Input: part model. Units: mm. Frame: model coordinates. A direction names the side the tool comes from. Give positions to 0.01 mm unless a question says otherwise; leave off trailing zeros. Order: outer loops, then holes, each group sorted by start corner. A loop starts at its lowest first (then second) coordinate and runs counter-clockwise, first axis right, second up. Notation, with made-up numbers: (0.25, -17.75) - (11.25, -17.75) arc R11 cw to (11.25, -4.75) - close; hole circle Ø11 at (-13.5, 57.5). An arc over 180 degrees is marked (long way). Answer in a Markdown table with one row per item. Add a question column.
1. Contact query for flat-ended pins moving along their axis: pin 1 (0.6 mm diameter, centred on y = 0, z = -7.5, fed in from +X); pin 2 (1.5 mm diameter, centred on x = 14.5, y = 0, fed in from -Z); pin 3 (0.9 mm diameter, centred on y = 0.5, z = -8, fed in from -X). Output: stop coordinate, or through.
2. Ray query, line 1 (X direction, y = 0.2, z = 11); line 2 (X direction, y = -0.25, z = -9); line 3 (Z direction, x = 16, y = 1.5). Return the intervals inside material, ascending. Write a range as [from, to].
3. Section query A-A on x = 0. Return loops of the section in (y, z).
4. Section query C-C on z = 9.75. Return loops of the section in (x, y).
5. Section query B-B on z = -2.25. Return loops of the section in (x, y), and give its area (3 significant figures).
6. Access query for faces 1 (the face through (20.237, 0, 3)), 2 (the face through (15, 0, -6.915)), 3 (the face through (-10.193, 0, -8)). Directions: +Z, -Z, +X, -X, +Y, -Y. A direction counts if a zero-diameter tool reaches every point of the face in a straight line with its end or side. Return the directions, or none.
7. Section query D-D on x = -13. Return loops of the section in (y, z).
8. Mould query, pull axis X, two halves, no side actions, for faces 4 (the face through (13.72, -0.04, 10.31)), 5 (the face through (-10.743, -0.035, 10.451)), 6 (the face through (-15, 0, -7.195)), 7 (the face through (10.237, 0, -8)). Classes: released by +X, released by -X, zero draft, split by the parting line, or undercut.
```python
from build123d import *

# Parameters (mm, degrees)
CROQUIS1_R              = 9.8
CROQUIS1_R_2            = 1.61
CROQUIS1_R_3            = 1.610199264
CROQUIS1_R_4            = 1.610298895
SALIENTE_EXTRUIR3_DEPTH = 2.5
REDONDEO1_SIZE          = 3
REDONDEO2_SIZE          = 3


with BuildPart() as part:
    # Croquis1 → Saliente-Extruir3 (new, symmetric)
    with BuildSketch(Plane(origin=(0, 0, 0), x_dir=(1, 0, 0), z_dir=(0, 1, 0))):
        Polygon((-20.192989013, 7.194690523), (-10.192989013, 7.194690523), (-10.192989013, 11.914690523), (10.237010987, 11.914690523), (10.237010987, 6.914690523), (20.237010987, 6.914690523), (20.237010987, -12.805309477), (-20.192989013, -12.805309477), align=None)
        with Locations(Location((0, -1.965309477, 0), (0, 0, 270))):
            Circle(CROQUIS1_R, mode=Mode.SUBTRACT)
        with Locations(Location((-12.339891833, 5.049690523, 0), (0, 0, 270))):
            Circle(CROQUIS1_R_2, mode=Mode.SUBTRACT)
        with Locations(Location((-12.339891833, -10.660508741, 0), (0, 0, 270))):
            Circle(CROQUIS1_R_3, mode=Mode.SUBTRACT)
        with Locations(Location((15.290108167, 5.049690523, 0), (0, 0, 270))):
            Circle(CROQUIS1_R_2, mode=Mode.SUBTRACT)
        with Locations(Location((15.290108167, -10.660608373, 0), (0, 0, 270))):
            Circle(CROQUIS1_R_4, mode=Mode.SUBTRACT)
        with Locations(Location((-7.653762012, 9.553535498, 0), (0, 0, 270))):
            Circle(CROQUIS1_R_4, mode=Mode.SUBTRACT)
        with Locations(Location((7.645768396, 9.553535498, 0), (0, 0, 270))):
            Circle(CROQUIS1_R_4, mode=Mode.SUBTRACT)
    extrude(amount=SALIENTE_EXTRUIR3_DEPTH, both=True)

    # Redondeo1
    # a fillet whose section is not a circle: 3 mm, written as the material it takes off along each edge
    with BuildSketch(Plane(origin=(10.237010987, 10, -11.914690523), x_dir=(0, 0, 1), z_dir=(0, -1, 0))) as redondeo1_piece_1:
        with BuildLine():
            add(Edge.make_bspline([(REDONDEO1_SIZE, 0), (REDONDEO1_SIZE * 0.831801948466, 0), (REDONDEO1_SIZE * 0.663603896932, 0), (REDONDEO1_SIZE * 0.292893218813, REDONDEO1_SIZE * 0.0716919198361), (REDONDEO1_SIZE * 0.0716919198361, REDONDEO1_SIZE * 0.292893218813), (0, REDONDEO1_SIZE * 0.663603896932), (0, REDONDEO1_SIZE * 0.831801948466), (0, REDONDEO1_SIZE)], knots=[0, 0, 0, 0, 0, 0, 0.5, 0.5, 1, 1, 1, 1, 1, 1], degree=5))
            Line((0, REDONDEO1_SIZE), (0, 0))
            Line((0, 0), (REDONDEO1_SIZE, 0))
        make_face()
    extrude(amount=20, mode=Mode.SUBTRACT)

    # Redondeo2
    # a fillet whose section is not a circle: 3 mm, written as the material it takes off along each edge
    with BuildSketch(Plane(origin=(-10.192989013, 10, -11.914690523), x_dir=(0, 0, 1), z_dir=(0, -1, 0))) as redondeo2_piece_1:
        with BuildLine():
            add(Edge.make_bspline([(REDONDEO2_SIZE, 0), (REDONDEO2_SIZE * 0.831801948466, 0), (REDONDEO2_SIZE * 0.663603896932, 0), (REDONDEO2_SIZE * 0.292893218813, -REDONDEO2_SIZE * 0.0716919198361), (REDONDEO2_SIZE * 0.0716919198361, -REDONDEO2_SIZE * 0.292893218813), (0, -REDONDEO2_SIZE * 0.663603896932), (0, -REDONDEO2_SIZE * 0.831801948466), (0, -REDONDEO2_SIZE)], knots=[0, 0, 0, 0, 0, 0, 0.5, 0.5, 1, 1, 1, 1, 1, 1], degree=5))
            Line((0, -REDONDEO2_SIZE), (0, 0))
            Line((0, 0), (REDONDEO2_SIZE, 0))
        make_face()
    extrude(amount=20, mode=Mode.SUBTRACT)


solid = part.part
```
Answer:
| question | item | result |
|---|---|---|
| 1 | pin 1 | stops at x = 10.24 |
| 1 | pin 2 | stops at z = -6.91 |
| 1 | pin 3 | stops at x = -10.19 |
| 2 | line 1 | x = [-20.19, -13.91], [-10.77, -3.8], [3.8, 13.72], [16.86, 20.24] |
| 2 | line 2 | x = [-10.19, -9.17], [-6.14, 6.13], [9.16, 10.24] |
| 2 | line 3 | z = [-6.91, -6.49], [-3.6, 9.22], [12.11, 12.81] |
| 3 | outline | (-2.5, -11.91) - (2.5, -11.91) - (2.5, -7.83) - (-2.5, -7.83) - close; (-2.5, 11.77) - (2.5, 11.77) - (2.5, 12.81) - (-2.5, 12.81) - close |
| 4 | outline | (-20.19, -2.5) - (-13.67, -2.5) - (-13.67, 2.5) - (-20.19, 2.5) - close; (-11.01, -2.5) - (-5.95, -2.5) - (-5.95, 2.5) - (-11.01, 2.5) - close; (5.95, -2.5) - (13.96, -2.5) - (13.96, 2.5) - (5.95, 2.5) - close; (16.62, -2.5) - (20.24, -2.5) - (20.24, 2.5) - (16.62, 2.5) - close |
| 5 | outline | (-20.19, -2.5) - (-8.85, -2.5) - (-8.85, 2.5) - (-20.19, 2.5) - close; (8.85, -2.5) - (20.24, -2.5) - (20.24, 2.5) - (8.85, 2.5) - close |
| 5 | area | 114 mm² |
| 6 | face 1 | +Z, -Z, +X, +Y, -Y |
| 6 | face 2 | -Z, +X, +Y, -Y |
| 6 | face 3 | -Z, -X, +Y, -Y |
| 7 | outline | (-2.5, -7.19) - (2.5, -7.19) - (2.5, -6.52) - (-2.5, -6.52) - close; (-2.5, -3.58) - (2.5, -3.58) - (2.5, 9.19) - (-2.5, 9.19) - close; (-2.5, 12.13) - (2.5, 12.13) - (2.5, 12.81) - (-2.5, 12.81) - close |
| 8 | face 4 | undercut |
| 8 | face 5 | undercut |
| 8 | face 6 | zero draft |
| 8 | face 7 | released by +X |
